Read the model definition and answer for the solid it produces. Units are mm, in the model's axes. A direction names the side the tool comes from. Coordinates: 2 decimals unless noted, no trailing zeros. Loops run counter-clockwise (first coordinate to the right, second up) from the corner with the lowest first, then second, coordinate; pieces in that order, holes last.
from build123d import *

# Parameters (mm, degrees)
SKETCH_2_R      = 1.5
EXTRUDE_3_DEPTH = 4
FILLET_2_R      = 3


with BuildPart() as part:
    # 草图2 → 凸台-拉伸3 (new body)
    with BuildSketch(Plane.XY):
        with BuildLine():
            Line((66.624685503, 252.532138716), (-83.375314497, 252.532138716))
            Line((-83.375314497, 252.532138716), (-83.375314497, 134.732138716))
            Line((-83.375314497, 134.732138716), (54.944685503, 134.732138716))
            Line((54.944685503, 134.732138716), (54.944685503, 152.232138716))
            ThreePointArc((54.944685503, 152.232138716), (53.18732619, 156.474779403), (48.944685503, 158.232138716))
            Line((48.944685503, 158.232138716), (27.544685503, 158.232138716))
            Line((27.544685503, 158.232138716), (27.544685503, 212.944120657))
            ThreePointArc((27.544685503, 212.944120657), (27.565107012, 213.229197834), (27.6259545, 213.508453305))
            Line((27.6259545, 213.508453305), (29.603509033, 220.232138716))
            Line((29.603509033, 220.232138716), (66.624685503, 220.232138716))
            Line((66.624685503, 220.232138716), (66.624685503, 252.532138716))
        make_face()
        with Locations((-30.875314497, 139.732138716)):
            Circle(SKETCH_2_R, mode=Mode.SUBTRACT)
        with Locations((-30.875314497, 149.732138716)):
            Circle(SKETCH_2_R, mode=Mode.SUBTRACT)
        with Locations((21.124685503, 173.232138716)):
            Circle(SKETCH_2_R, mode=Mode.SUBTRACT)
        with Locations((21.124685503, 203.232138716)):
            Circle(SKETCH_2_R, mode=Mode.SUBTRACT)
        with BuildLine():
            Line((18.644685503, 151.232138716), (25.644685503, 151.232138716))
            ThreePointArc((25.644685503, 151.232138716), (27.144685503, 149.732138716), (25.644685503, 148.232138716))
            Line((25.644685503, 148.232138716), (18.644685503, 148.232138716))
            ThreePointArc((18.644685503, 148.232138716), (17.144685503, 149.732138716), (18.644685503, 151.232138716))
        make_face(mode=Mode.SUBTRACT)
        with BuildLine():
            Line((25.644685503, 138.232138716), (18.644685503, 138.232138716))
            ThreePointArc((18.644685503, 138.232138716), (17.144685503, 139.732138716), (18.644685503, 141.232138716))
            Line((18.644685503, 141.232138716), (25.644685503, 141.232138716))
            ThreePointArc((25.644685503, 141.232138716), (27.144685503, 139.732138716), (25.644685503, 138.232138716))
        make_face(mode=Mode.SUBTRACT)
        with Locations((37.444685503, 223.232138716)):
            Circle(SKETCH_2_R, mode=Mode.SUBTRACT)
        with Locations((47.044685503, 149.732138716)):
            Circle(SKETCH_2_R, mode=Mode.SUBTRACT)
        with Locations((47.044685503, 139.732138716)):
            Circle(SKETCH_2_R, mode=Mode.SUBTRACT)
    extrude(amount=EXTRUDE_3_DEPTH)

    # 圆角2
    fillet_2_edges = [part.edges().sort_by_distance(p)[0] for p in [
        (-83.375314497, 134.732138716, 2),
        (-83.375314497, 252.532138716, 2),
        (66.624685503, 252.532138716, 2),
        (66.624685503, 220.232138716, 2),
        (54.944685503, 134.732138716, 2),
    ]]
    fillet(fillet_2_edges, radius=FILLET_2_R)


solid = part.part
Item 1: A cutting plane is placed at C-C on y = 146. Determine the outline of the cut face in (x, z), then the cut area to 3 significant figures.
Numbers:
outline: (-83.38, 0) - (54.94, 0) - (54.94, 4) - (-83.38, 4) - close
area: 553 mm2
Item 2: Given pin 1 (2 mm diameter, centred on y = 143, z = 2, fed in from +X); pin 2 (1.8 mm diameter, centred on x = 47.04, y = 139.73, fed in from +Z), each flat-ended and moving along its own axis, determine where each tip first touches the part or whether it passes through.
Numbers:
pin 1: stops at x = 54.94
pin 2: passes through
Item 3: A cutting plane is placed at B-B on y = 200. Determine the outline of the cut face in (x, z).
Numbers:
outline: (-83.38, 0) - (27.54, 0) - (27.54, 4) - (-83.38, 4) - close
Item 4: Which of the six approach directions +Z, -Z, +X, -X, +Y, -Y give full straight-line access (tool end or side, diameter ignored) to faces 1 (the face through (66.625, 236, 2)), 2 (the face through (27.144, 149.765, 1.972)), 3 (the face through (46, 220.232, 2)), 4 (the face through (54.945, 145, 2)), 5 (the face through (-82.52, 135.634, 2.028))?
Numbers:
face 1: +Z, -Z, +X, +Y, -Y
face 2: +Z, -Z
face 3: +Z, -Z, +X
face 4: +Z, -Z, +X, -Y
face 5: +Z, -Z, -X, -Y
Item 5: A cutting plane is placed at A-A on z = 1.1. Give the number of separate pieces and of enclosed holes in the cut face, then the cut area to 3 significant figures.
Numbers:
separate pieces: 1
enclosed holes: 9
area: 14,900 mm2
Item 6: Determine the mould class of faces 6 (the face through (-32.374, 149.798, 1.972)), 7 (the face through (38, 158.232, 2)), 8 (the face through (45.546, 149.798, 1.972)), 9 (the face through (53.23, 156.43, 1.97)) for opening direction X: released by +X, released by -X, zero draft, split by the parting line, or undercut.
Numbers:
face 6: undercut
face 7: zero draft
face 8: undercut
face 9: released by +X
Item 7: Find the intervals of material crossed by line 1 along X through (y, z) = (149.5, 1.9); line 2 along Y through (x, z) = (24, 3.55); line 3 along Y through (x, z) = (37, 2.7), in increasing order.
Numbers:
line 1: x = -83.38 to -32.36, -29.39 to 17.16, 27.13 to 45.56, 48.53 to 54.94
line 2: y = 134.73 to 138.23, 141.23 to 148.23, 151.23 to 252.53
line 3: y = 134.73 to 158.23, 220.23 to 221.8, 224.66 to 252.53
